The model under review builds one solid part; all positions refer to its coordinate system, in mm. Face numbers are marked on the shaded views. Coordinates: 2 decimals unless noted, no trailing zeros. Write each loop counter-clockwise with the first axis right and the second up, starting at its lowest first coordinate (ties: lowest second). Pieces come first, ordered by that corner, then holes.
1) Add section A-A, the plane x = 0. State the section outline as (y, z) points, then the cut area to 3 significant figures.
2) For line 1 (X direction, y = 3.5, z = 0); line 2 (Y direction, x = 24, z = -5.5); line 3 (Z direction, x = 2.5, y = 7.25), list the stretches that pass through material, from the lowest coordinate up.
3) Add section C-C, the plane y = 1.5. State the section outline as (x, z) points.
4) Add section B-B, the plane z = 0. State the section outline as (x, y) points.
5) Add section D-D, the plane x = -20. State the section outline as (y, z) points.
6) For P1, Ø4, axis at x = -24, y = 7.5, coming from the +Z side; P2, Ø17, axis at x = 0, z = 0, coming from the +Y side; P3, Ø5, axis at x = 23.5, y = 4, coming from the -Z side; P4, Ø4, axis at x = -22, z = 38, coming from the -Y side, all flat-tipped, find the tip position at first contact; note any pin that passes through.
7) Mouldability with a two-part tool opening along Z and no side actions: class the marked faces 1, 2 and 3 as released by +Z, released by -Z, zero draft, split by the parting line, or undercut.
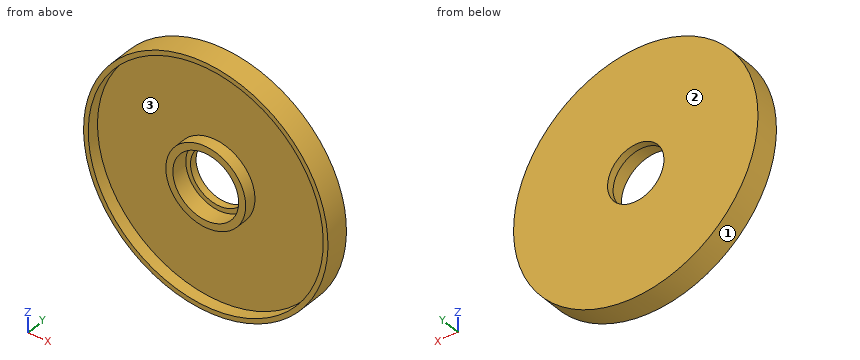
from build123d import *

# Parameters (mm, degrees)
SKETCH1_R           = 52
BOSS_EXTRUDE1_DEPTH = 10
SKETCH2_R           = 50
CUT_EXTRUDE4_DEPTH  = 5
SKETCH3_R           = 12
CUT_EXTRUDE7_DEPTH  = 10
SKETCH4_R           = 17
BOSS_EXTRUDE2_DEPTH = 5
SKETCH5_R           = 14
CUT_EXTRUDE8_DEPTH  = 7


with BuildPart() as part:
    # Sketch1 → Boss-Extrude1 (new body)
    with BuildSketch(Plane(origin=(0, 0, 0), x_dir=(1, 0, 0), z_dir=(0, 1, 0))):
        with Locations(Location((0, 0, 0), (0, 0, 270))):
            Circle(SKETCH1_R)
    extrude(amount=BOSS_EXTRUDE1_DEPTH)

    # Sketch2 → Cut-Extrude4 (cut)
    with BuildSketch(Plane(origin=(0, 0, 0), x_dir=(1, 0, 0), z_dir=(0, 1, 0))):
        with Locations(Location((0, 0, 0), (0, 0, 270))):
            Circle(SKETCH2_R)
    extrude(amount=CUT_EXTRUDE4_DEPTH, mode=Mode.SUBTRACT)

    # Sketch3 → Cut-Extrude7 (cut)
    with BuildSketch(Plane(origin=(0, 0, 0), x_dir=(1, 0, 0), z_dir=(0, 1, 0))):
        with Locations(Location((0, 0, 0), (0, 0, 270))):
            Circle(SKETCH3_R)
    extrude(amount=CUT_EXTRUDE7_DEPTH, mode=Mode.SUBTRACT)

    # Sketch4 → Boss-Extrude2 (add)
    with BuildSketch(Plane.XZ.offset(-5)):
        with Locations(Location((0, 0, 0), (0, 0, 90))):
            Circle(SKETCH4_R)
    extrude(amount=BOSS_EXTRUDE2_DEPTH)

    # Sketch5 → Cut-Extrude8 (cut)
    with BuildSketch(Plane.XZ):
        with Locations(Location((0, 0, 0), (0, 0, 270))):
            Circle(SKETCH5_R)
    extrude(amount=-CUT_EXTRUDE8_DEPTH, mode=Mode.SUBTRACT)


solid = part.part
Geometry results:
1. outline: (0, -52) - (10, -52) - (10, -12) - (7, -12) - (7, -14) - (0, -14) - (0, -17) - (5, -17) - (5, -50) - (0, -50) - close; (0, 14) - (7, 14) - (7, 12) - (10, 12) - (10, 52) - (0, 52) - (0, 50) - (5, 50) - (5, 17) - (0, 17) - close
1. area: 442 mm2
2. line 1: x = -52 to -50, -17 to -14, 14 to 17, 50 to 52
2. line 2: y = 5 to 10
2. line 3: z = -51.94 to -11.74, 11.74 to 51.94
3. outline: circle Ø104 at (0, 0); circle Ø34 at (0, 0); hole circle Ø100 at (0, 0); hole circle Ø28 at (0, 0)
4. outline: (-52, 0) - (-50, 0) - (-50, 5) - (-17, 5) - (-17, 0) - (-14, 0) - (-14, 7) - (-12, 7) - (-12, 10) - (-52, 10) - close; (12, 7) - (14, 7) - (14, 0) - (17, 0) - (17, 5) - (50, 5) - (50, 0) - (52, 0) - (52, 10) - (12, 10) - close
5. outline: (0, -48) - (10, -48) - (10, 48) - (0, 48) - (0, 45.83) - (5, 45.83) - (5, -45.83) - (0, -45.83) - close
6. P1: stops at z = 47.12
6. P2: passes through
6. P3: stops at z = -47.57
6. P4: stops at y = 5
7. face 1: split by the parting line
7. face 2: zero draft
7. face 3: undercut
